Verification items for the finished model (mm, model axes). A direction names the side the tool comes from. Give positions to 0.01 mm unless a question says otherwise; leave off trailing zeros. Write each loop counter-clockwise with the first axis right and the second up, starting at its lowest first coordinate (ties: lowest second). Pieces come first, ordered by that corner, then holes. Notation, with made-up numbers: M -16.5,58.25 L 3.5,58.25 A20 cw 3.5,74.25 Z; hole C 31.25,54 d5. An arc over 180 degrees is marked long. Write item = value, one per line.
from build123d import *

# Parameters (mm, degrees)
SKETCH1_W             = 38.1
SKETCH1_H             = 63.5
BOSS_EXTRUDE1_DEPTH   = 3.175
F_4_CLEARANCE_HOLE1_D = 3.2639
CUT_EXTRUDE3_REACH    = 76.325
SKETCH6_W             = 12.7
SKETCH6_H             = 6.35
CUT_EXTRUDE4_REACH    = 76.325
SKETCH10_W            = 15.494
SKETCH10_H            = 15.621
LPATTERN1_COUNT       = 2
LPATTERN1_PITCH       = 22.225
FILLET1_R             = 0.508


with BuildPart() as part:
    # Sketch1 → Boss-Extrude1 (new, symmetric)
    with BuildSketch(Plane.XY):
        with Locations((19.05, -31.75)):
            Rectangle(SKETCH1_W, SKETCH1_H)
    extrude(amount=BOSS_EXTRUDE1_DEPTH, both=True)

    # #4 Clearance Hole1 (through all)
    with Locations(Plane.XY.offset(3.175)):
        with Locations((6.35, -3.175), (31.75, -3.175)):
            Hole(F_4_CLEARANCE_HOLE1_D / 2)

    # Sketch6 → Cut-Extrude3 (cut, up to next)
    with BuildSketch(Plane.XY.offset(3.175), mode=Mode.PRIVATE) as cut_extrude3_sk1:
        with Locations((19.05, -3.175)):
            Rectangle(SKETCH6_W, SKETCH6_H)
    cut_extrude3_tool1 = extrude(cut_extrude3_sk1.sketch, amount=-CUT_EXTRUDE3_REACH, mode=Mode.PRIVATE) & part.part
    add(cut_extrude3_tool1.solids().sort_by_distance((19.05, -3.175, 3.175))[0], mode=Mode.SUBTRACT)

    # Sketch10 → Cut-Extrude4 (cut, up to next)
    with BuildSketch(Plane(origin=(0, 0, -3.175), x_dir=(-1, 0, 0), z_dir=(0, 0, -1)), mode=Mode.PRIVATE) as cut_extrude4_sk1:
        with Locations((-19.05, -26.9875)):
            Rectangle(SKETCH10_W, SKETCH10_H)
    cut_extrude4_tool1 = extrude(cut_extrude4_sk1.sketch, amount=-CUT_EXTRUDE4_REACH, mode=Mode.PRIVATE) & part.part
    cut_extrude4 = cut_extrude4_tool1.solids().sort_by_distance((19.05, -26.9875, -3.175))[0]
    add(cut_extrude4, mode=Mode.SUBTRACT)

    # LPattern1: Cut-Extrude4 ×2
    with Locations(*[(0, -i * LPATTERN1_PITCH, 0) for i in range(1, LPATTERN1_COUNT)]):
        add(cut_extrude4, mode=Mode.SUBTRACT)

    # Fillet1
    fillet1_edges = [part.edges().sort_by_distance(p)[0] for p in [
        (11.303, -19.177, 0),
        (11.303, -34.798, 0),
        (26.797, -34.798, 0),
        (26.797, -19.177, 0),
        (11.303, -41.402, 0),
        (11.303, -57.023, 0),
        (26.797, -57.023, 0),
        (26.797, -41.402, 0),
    ]]
    fillet(fillet1_edges, radius=FILLET1_R)


solid = part.part
1) Cross-section at D-D on x = 18. Record the boundary of the cut face in (y, z) (3 decimals).
From the geometry:
outline = M -63.5,-3.175 L -57.023,-3.175 L -57.023,3.175 L -63.5,3.175 Z; M -41.402,-3.175 L -34.798,-3.175 L -34.798,3.175 L -41.402,3.175 Z; M -19.177,-3.175 L -6.35,-3.175 L -6.35,3.175 L -19.177,3.175 Z
2) Cross-section at B-B on x = 31.75. Record the boundary of the cut face in (y, z) (3 decimals).
From the geometry:
outline = M -63.5,-3.175 L -4.807,-3.175 L -4.807,3.175 L -63.5,3.175 Z; M -1.543,-3.175 L 0,-3.175 L 0,3.175 L -1.543,3.175 Z
3) Depth check by flat-ended pin: P1, Ø1.9, axis at x = 21.5, z = -0.5, coming from the +Y side. Enter the tip coordinate at first touch or a pass-through.
From the geometry:
P1 = -6.35
4) Cross-section at C-C on z = -1.5. Record the boundary of the cut face in (x, y) (3 decimals).
From the geometry:
outline = M 0,-63.5 L 38.1,-63.5 L 38.1,0 L 25.4,0 L 25.4,-6.35 L 12.7,-6.35 L 12.7,0 L 0,0 Z; hole C 6.35,-3.175 d3.264; hole M 11.303,-56.515 A0.508 ccw 11.811,-57.023 L 26.289,-57.023 A0.508 ccw 26.797,-56.515 L 26.797,-41.91 A0.508 ccw 26.289,-41.402 L 11.811,-41.402 A0.508 ccw 11.303,-41.91 Z; hole M 11.303,-34.29 A0.508 ccw 11.811,-34.798 L 26.289,-34.798 A0.508 ccw 26.797,-34.29 L 26.797,-19.685 A0.508 ccw 26.289,-19.177 L 11.811,-19.177 A0.508 ccw 11.303,-19.685 Z; hole C 31.75,-3.175 d3.264
5) Draft check along Y on faces 1 (the flat face through (12.7, -3, 0)), 2 (the flat face through (19, -6.35, 0)), 3 (the cylindrical face through (7.645, -4.168, -0.044)). Enter one of: +Y half, -Y half, draft (parallel to the pull), parting line (faces both ways), or undercut.
From the geometry:
face_1 = draft
face_2 = +Y half
face_3 = undercut
6) Cross-section at A-A on y = -20.5. Record the boundary of the cut face in (x, z) (3 decimals), plus the area to 3 significant figures.
From the geometry:
outline = M 0,-3.175 L 11.303,-3.175 L 11.303,3.175 L 0,3.175 Z; M 26.797,-3.175 L 38.1,-3.175 L 38.1,3.175 L 26.797,3.175 Z
area = 144 mm^2
7) Tool access check on faces 4 (the flat face through (6, 0, 0)), 5 (the flat face through (19, -19.177, 0)), 6 (the flat face through (25.4, -3, 0)). Record the directions out of +Z, -Z, +X, -X, +Y, -Y that give a thin tool (end or side, any length) a straight path to the whole face; none if there is none.
From the geometry:
face_4 = +Z, -Z, +X, -X, +Y
face_5 = +Z, -Z
face_6 = +Z, -Z, +Y
8) Material ranges on probe 1 along Y at (x, z) = (19, -0.75); probe 2 along Y at (x, z) = (12.5, -1.5); probe 3 along Y at (x, z) = (6.35, -1.5), recorded low to high. Write a range as from..to.
From the geometry:
probe_1 = -63.5..-57.02, -41.4..-34.8, -19.18..-6.35
probe_2 = -63.5..-57.02, -41.4..-34.8, -19.18..0
probe_3 = -63.5..-4.81, -1.54..0
